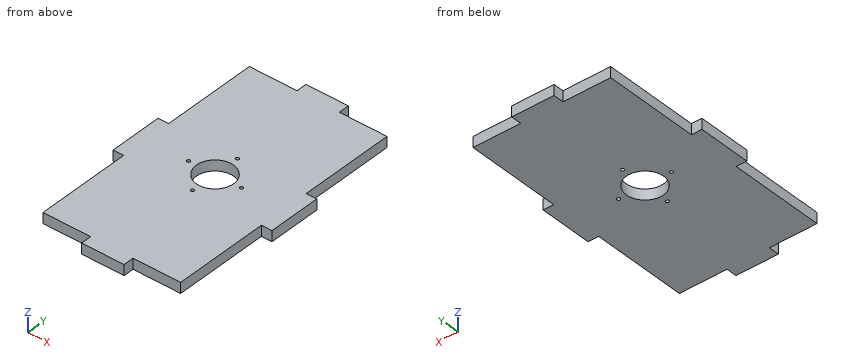
Autodesk Fusion 360 part; units mm, degrees
sketch "Esquisse1" plane through (0, 0, 0) normal (0, 0, 1) x (1, 0, 0)
  line L0 (75, -125) -> (-75, -125) construction
  line L1 (-75, -125) -> (-75, 125) construction
  line L2 (-75, 125) -> (75, 125) construction
  line L3 (75, 125) -> (75, -125) construction
  line L4 (75, -125) -> (-75, 125) construction
  line L5 (-75, -125) -> (75, 125) construction
  circle A0 centre (0, 0) radius 17.5
  circle A1 centre (0, 0) radius 25 construction
  circle A2 centre (0, 25) radius 1.6
  circle A3 centre (-25, 0) radius 1.6
  circle A4 centre (0, -25) radius 1.6
  circle A5 centre (25, 0) radius 1.6
  line L6 (0, 125) -> (0, -125)
  line L7 (-75, 0) -> (75, 0)
  line L8 (75, 125) -> (-75, 125) construction
  line L9 (-75, -125) -> (75, -125) construction
  line L10 (75, -125) -> (-75, -125) construction
  line L11 (-65, 115) -> (-65, 25)
  line L12 (-65, 25) -> (-75, 25)
  line L13 (-75, 25) -> (-75, -25)
  line L14 (-75, -25) -> (-65, -25)
  line L15 (-65, -25) -> (-65, -115)
  line L16 (65, 115) -> (65, 25)
  line L17 (65, 25) -> (75, 25)
  line L18 (75, -125) -> (75, 125) construction
  line L19 (75, -25) -> (65, -25)
  line L20 (65, -25) -> (65, -115)
  line L21 (75, 25) -> (75, -25)
  line L22 (-65, 115) -> (-20, 115)
  line L23 (-20, 115) -> (-20, 125)
  line L24 (20, 125) -> (-20, 125)
  line L25 (20, 125) -> (20, 115)
  line L26 (20, 115) -> (65, 115)
  line L27 (20, -125) -> (20, -115)
  line L28 (20, -115) -> (65, -115)
  line L29 (20, -125) -> (-20, -125)
  line L30 (-20, -115) -> (-20, -125)
  line L31 (-65, -115) -> (-20, -115)
  circle A6 centre (0, 0) radius 33.25 construction
  dimension "d1" = 150
  dimension "d2" = 250
  dimension "d3" = 35
  dimension "d5" = 3.2
  dimension "d9" = 50
  dimension "d14" = 40
  dimension "d15" = 10
  dimension "d16" = 10
  dimension "d17" = 66.5
  dimension "d18" = 50
  dimension "d25" = 10
extrude "Extrusion1" add sketch "Esquisse1" along normal blind 10 contours A0 A4 A5 L6 L7 L19 L20 L21 L27 L28 L29 | A0 A2 A5 L6 L7 L16 L17 L21 L24 L25 L26 | A0 A2 A3 L6 L7 L11 L12 L13 L22 L23 L24 | A0 A3 A4 L6 L7 L13 L14 L15 L29 L30 L31
Source: CAD feature listing. Evaluate the final solid. Frame: model axes, mm. Round coordinates to 2 decimals unless told otherwise and drop trailing zeros. Write each loop counter-clockwise with the first axis right and the second up, starting at its lowest first coordinate (ties: lowest second). Pieces come first, ordered by that corner, then holes. Notation, with made-up numbers: M 62,53 L 83,53 A38 ccw 83,92 Z; hole C 28,71 d4. An arc over 180 degrees is marked long. One line per item, written item: value. Start each with the question number.
Item 1: Ray query, L1, parallel to X at y = 0, z = 5.25; L2, parallel to Y at x = 0, z = 5; L3, parallel to Y at x = -25, z = 7.25. Return the intervals inside material, ascending. Write a range as from..to.
Item 2: Section query A-A (z = 7). Return the cut outline in (x, y), plus the area to 3 significant figures.
Item 3: Pin query (flat end, axial travel): pin 1 (5 mm diameter, centred on x = 70, z = 6, fed in from -Y); pin 2 (1 mm diameter, centred on x = -53, z = 1.5, fed in from +Y); pin 3 (3 mm diameter, centred on y = 119, z = 3.5, fed in from +X); pin 4 (1.9 mm diameter, centred on x = -25, y = 0, fed in from +Z). Return the tip coordinate at first contact, or that it passes through.
Item 4: Section query D-D (y = -101). Return the cut outline in (x, z), plus the area to 3 significant figures.
Item 5: Section query C-C (x = -15). Return the cut outline in (y, z).
Item 6: Section query B-B (y = 11.5). Return the cut outline in (x, z), plus the area to 3 significant figures.
Result set:
1. L1: x = -75..-26.6, -23.4..-17.5, 17.5..23.4, 26.6..75
1. L2: y = -125..-26.6, -23.4..-17.5, 17.5..23.4, 26.6..125
1. L3: y = -115..-1.6, 1.6..115
2. outline: M -75,-25 L -65,-25 L -65,-115 L -20,-115 L -20,-125 L 20,-125 L 20,-115 L 65,-115 L 65,-25 L 75,-25 L 75,25 L 65,25 L 65,115 L 20,115 L 20,125 L -20,125 L -20,115 L -65,115 L -65,25 L -75,25 Z; hole C -25,0 d3.2; hole C 0,0 d35; hole C 0,-25 d3.2; hole C 0,25 d3.2; hole C 25,0 d3.2
2. area: 30,700 mm²
3. pin 1: stops at y = -25
3. pin 2: stops at y = 115
3. pin 3: stops at x = 20
3. pin 4: passes through
4. outline: M -65,0 L 65,0 L 65,10 L -65,10 Z
4. area: 1,300 mm²
5. outline: M -125,0 L -9.01,0 L -9.01,10 L -125,10 Z; M 9.01,0 L 125,0 L 125,10 L 9.01,10 Z
6. outline: M -75,0 L -13.19,0 L -13.19,10 L -75,10 Z; M 13.19,0 L 75,0 L 75,10 L 13.19,10 Z
6. area: 1,240 mm²
